Verification items for the finished model (mm, model axes). Face numbers are marked on the shaded views. A direction names the side the tool comes from. Coordinates: 2 decimals unless noted, no trailing zeros. Write each loop counter-clockwise with the first axis right and the second up, starting at its lowest first coordinate (ties: lowest second). Pieces come first, ordered by that corner, then holes. Notation, with made-up numbers: (-25, 23.25) - (28, 23.25) arc R26 ccw to (28, 62.25) - close; hole circle Ø2 at (14, 80). An arc over 180 degrees is marked (long way). Use CSV: the item, a comma, the result in double quotes. Start each with the question number.
```python
from build123d import *

# Parameters (mm, degrees)
F3_W          = 60
F3_H          = 91
F4_DEPTH      = 10
F5_W          = 56
F5_H          = 87
F6_DEPTH      = 8
F7_R          = 4
F8_DEPTH      = 10
F9_R          = 2
F10_DEPTH     = 10.001
F11_R         = 5
F12_R         = 5
F13_T1_DEPTH  = 77
F13_T3_DEPTH  = 14.5147186258
F13_T5_DEPTH  = 14.5147186258
F13_T8_ANGLE  = 90
F13_T10_ANGLE = 70.5287793655
F13_T12_ANGLE = 141.057558731
F13_T14_ANGLE = 90
F13_T16_ANGLE = 70.5287793655
F13_T18_ANGLE = 70.5287793655
F13_T20_ANGLE = 90
F13_T22_ANGLE = 141.057558731
F13_T24_ANGLE = 70.5287793655
F13_T26_ANGLE = 90
F13_T27_DEPTH = 81
F13_T29_DEPTH = 50
F13_T32_ANGLE = 90
F13_T34_ANGLE = 90
F13_T36_ANGLE = 90
F13_T38_ANGLE = 90


# Not quite as in the source:
# - a fillet or chamfer that OpenCascade refuses, or shapes differently, is made with other operations: its cross-section is extruded or revolved along the edge and cut away or added


with BuildPart() as f4:
    # F3 (on Top) → F4 (new body)
    with BuildSketch(Plane.XY):
        Rectangle(F3_W, F3_H)
    extrude(amount=F4_DEPTH)

    # F5 (on face) → F6 (cut)
    with BuildSketch(Plane.XY.offset(10)):
        Rectangle(F5_W, F5_H)
    extrude(amount=-F6_DEPTH, mode=Mode.SUBTRACT)

    # F7 (on face) → F8 (join)
    with BuildSketch(Plane(origin=(0, 0, 0), x_dir=(1, 0, 0), z_dir=(0, 0, -1))):
        with Locations((0, -41.5)):
            Circle(F7_R)
        with Locations((0, 41.5)):
            Circle(F7_R)
    extrude(amount=-F8_DEPTH)

    # F9 (on face) → F10 (cut, through all)
    with BuildSketch(Plane(origin=(0, 0, 0), x_dir=(1, 0, 0), z_dir=(0, 0, -1))):
        with Locations((0, -41.5)):
            Circle(F9_R)
        with Locations((0, 41.5)):
            Circle(F9_R)
    extrude(amount=-F10_DEPTH, mode=Mode.SUBTRACT)

    # F11
    f11_edges = [f4.edges().sort_by_distance(p)[0] for p in [
        (3.464102, 43.5, 6),
        (-3.464102, 43.5, 6),
        (-3.464102, -43.5, 6),
        (3.464102, -43.5, 6),
    ]]
    fillet(f11_edges, radius=F11_R)

    # F12
    f12_edges = [f4.edges().sort_by_distance(p)[0] for p in [
        (30, -45.5, 5),
        (-30, -45.5, 5),
        (30, 45.5, 5),
        (-30, 45.5, 5),
        (28, -43.5, 6),
        (-28, -43.5, 6),
        (-28, 43.5, 6),
        (28, 43.5, 6),
    ]]
    fillet(f12_edges, radius=F12_R)

    # F13: fillet of radius 3 on 24 edges, made by hand

    # F13_s2 → F13_t1 (join)
    with BuildSketch(Plane.XZ.offset(-38.5)):
        with BuildLine():
            ThreePointArc((-28, 5), (-27.1213203436, 2.8786796564), (-25, 2))
            Line((-25, 2), (-28, 2))
            Line((-28, 2), (-28, 5))
        make_face()
        with BuildLine():
            ThreePointArc((28, 5), (27.1213203436, 2.8786796564), (25, 2))
            Line((25, 2), (28, 2))
            Line((28, 2), (28, 5))
        make_face()
    extrude(amount=F13_T1_DEPTH)

    # F13_s4 → F13_t3 (join)
    with BuildSketch(Plane.YZ.offset(8.4852813742)):
        with BuildLine():
            ThreePointArc((-43.5, 5), (-42.6213203436, 2.8786796564), (-40.5, 2))
            Line((-40.5, 2), (-43.5, 2))
            Line((-43.5, 2), (-43.5, 5))
        make_face()
        with BuildLine():
            ThreePointArc((43.5, 5), (42.6213203436, 2.8786796564), (40.5, 2))
            Line((40.5, 2), (43.5, 2))
            Line((43.5, 2), (43.5, 5))
        make_face()
    extrude(amount=F13_T3_DEPTH)

    # F13_s6 → F13_t5 (join)
    with BuildSketch(Plane.YZ.offset(-23)):
        with BuildLine():
            ThreePointArc((-43.5, 5), (-42.6213203436, 2.8786796564), (-40.5, 2))
            Line((-40.5, 2), (-43.5, 2))
            Line((-43.5, 2), (-43.5, 5))
        make_face()
        with BuildLine():
            ThreePointArc((43.5, 5), (42.6213203436, 2.8786796564), (40.5, 2))
            Line((40.5, 2), (43.5, 2))
            Line((43.5, 2), (43.5, 5))
        make_face()
    extrude(amount=F13_T5_DEPTH)

    # F13_s7 → F13_t8 (revolve)
    with BuildSketch(Plane.YZ.offset(23)):
        with BuildLine():
            ThreePointArc((-43.5, 5), (-42.6213203436, 2.8786796564), (-40.5, 2))
            Line((-40.5, 2), (-43.5, 2))
            Line((-43.5, 2), (-43.5, 5))
        make_face()
    revolve(axis=Axis((23, -38.5, 2), (0, 0, 1)), revolution_arc=F13_T8_ANGLE)

    # F13_s9 → F13_t10 (revolve)
    with BuildSketch(Plane.YZ.offset(8.4852813742)):
        with BuildLine():
            ThreePointArc((-43.5, 5), (-42.6213203436, 2.8786796564), (-40.5, 2))
            Line((-40.5, 2), (-43.5, 2))
            Line((-43.5, 2), (-43.5, 5))
        make_face()
    revolve(axis=Axis((8.4852813742, -38.5, 2), (0, 0, -1)), revolution_arc=F13_T10_ANGLE)

    # F13_s11 → F13_t12 (revolve)
    with BuildSketch(Plane(origin=(-13.0421917419, -36.8888888889, 0), x_dir=(0, 0, 1), z_dir=(-0.3333333333, -0.9428090416, 0))):
        with BuildLine():
            ThreePointArc((5, -9.8333333333), (2.8786796564, -8.9546536769), (2, -6.8333333333))
            Line((2, -6.8333333333), (2, -9.8333333333))
            Line((2, -9.8333333333), (5, -9.8333333333))
        make_face()
    revolve(axis=Axis((0, -41.5, 2), (0, 0, -1)), revolution_arc=F13_T12_ANGLE)

    # F13_s13 → F13_t14 (revolve)
    with BuildSketch(Plane.XZ.offset(-38.5)):
        with BuildLine():
            ThreePointArc((28, 5), (27.1213203436, 2.8786796564), (25, 2))
            Line((25, 2), (28, 2))
            Line((28, 2), (28, 5))
        make_face()
    revolve(axis=Axis((23, 38.5, 2), (0, 0, 1)), revolution_arc=F13_T14_ANGLE)

    # F13_s15 → F13_t16 (revolve)
    with BuildSketch(Plane(origin=(-13.0421917419, -36.8888888889, 0), x_dir=(0, 0, 1), z_dir=(0.3333333333, 0.9428090416, 0))):
        with BuildLine():
            ThreePointArc((5, 9.8333333333), (2.8786796564, 8.9546536769), (2, 6.8333333333))
            Line((2, 6.8333333333), (2, 9.8333333333))
            Line((2, 9.8333333333), (5, 9.8333333333))
        make_face()
    revolve(axis=Axis((-8.4852813742, -38.5, 2), (0, 0, -1)), revolution_arc=F13_T16_ANGLE)

    # F13_s17 → F13_t18 (revolve)
    with BuildSketch(Plane.YZ.offset(8.4852813742)):
        with BuildLine():
            ThreePointArc((43.5, 5), (42.6213203436, 2.8786796564), (40.5, 2))
            Line((40.5, 2), (43.5, 2))
            Line((43.5, 2), (43.5, 5))
        make_face()
    revolve(axis=Axis((8.4852813742, 38.5, 2), (0, 0, 1)), revolution_arc=F13_T18_ANGLE)

    # F13_s19 → F13_t20 (revolve)
    with BuildSketch(Plane.YZ.offset(-23)):
        with BuildLine():
            ThreePointArc((-43.5, 5), (-42.6213203436, 2.8786796564), (-40.5, 2))
            Line((-40.5, 2), (-43.5, 2))
            Line((-43.5, 2), (-43.5, 5))
        make_face()
    revolve(axis=Axis((-23, -38.5, 2), (0, 0, -1)), revolution_arc=F13_T20_ANGLE)

    # F13_s21 → F13_t22 (revolve)
    with BuildSketch(Plane(origin=(13.0421917419, 36.8888888889, 0), x_dir=(0, 0, 1), z_dir=(0.3333333333, 0.9428090416, 0))):
        with BuildLine():
            ThreePointArc((5, -9.8333333333), (2.8786796564, -8.9546536769), (2, -6.8333333333))
            Line((2, -6.8333333333), (2, -9.8333333333))
            Line((2, -9.8333333333), (5, -9.8333333333))
        make_face()
    revolve(axis=Axis((0, 41.5, 2), (0, 0, -1)), revolution_arc=F13_T22_ANGLE)

    # F13_s23 → F13_t24 (revolve)
    with BuildSketch(Plane(origin=(-13.0421917419, 36.8888888889, 0), x_dir=(0, 0, 1), z_dir=(0.3333333333, -0.9428090416, 0))):
        with BuildLine():
            ThreePointArc((5, -9.8333333333), (2.8786796564, -8.9546536769), (2, -6.8333333333))
            Line((2, -6.8333333333), (2, -9.8333333333))
            Line((2, -9.8333333333), (5, -9.8333333333))
        make_face()
    revolve(axis=Axis((-8.4852813742, 38.5, 2), (0, 0, 1)), revolution_arc=F13_T24_ANGLE)

    # F13_s25 → F13_t26 (revolve)
    with BuildSketch(Plane.XZ.offset(-38.5)):
        with BuildLine():
            ThreePointArc((-28, 5), (-27.1213203436, 2.8786796564), (-25, 2))
            Line((-25, 2), (-28, 2))
            Line((-28, 2), (-28, 5))
        make_face()
    revolve(axis=Axis((-23, 38.5, 2), (0, 0, -1)), revolution_arc=F13_T26_ANGLE)

    # F13_s28 → F13_t27 (cut)
    with BuildSketch(Plane.XZ.offset(-40.5)):
        with BuildLine():
            ThreePointArc((30, 3), (29.1213203436, 0.8786796564), (27, 0))
            Line((27, 0), (30, 0))
            Line((30, 0), (30, 3))
        make_face()
        with BuildLine():
            ThreePointArc((-30, 3), (-29.1213203436, 0.8786796564), (-27, 0))
            Line((-27, 0), (-30, 0))
            Line((-30, 0), (-30, 3))
        make_face()
    extrude(amount=F13_T27_DEPTH, mode=Mode.SUBTRACT)

    # F13_s30 → F13_t29 (cut)
    with BuildSketch(Plane.YZ.offset(-25)):
        with BuildLine():
            ThreePointArc((-45.5, 3), (-44.6213203436, 0.8786796564), (-42.5, 0))
            Line((-42.5, 0), (-45.5, 0))
            Line((-45.5, 0), (-45.5, 3))
        make_face()
        with BuildLine():
            ThreePointArc((45.5, 3), (44.6213203436, 0.8786796564), (42.5, 0))
            Line((42.5, 0), (45.5, 0))
            Line((45.5, 0), (45.5, 3))
        make_face()
    extrude(amount=F13_T29_DEPTH, mode=Mode.SUBTRACT)

    # F13_s31 → F13_t32 (revolve, cut)
    with BuildSketch(Plane.YZ.offset(25)):
        with BuildLine():
            ThreePointArc((-45.5, 3), (-44.6213203436, 0.8786796564), (-42.5, 0))
            Line((-42.5, 0), (-45.5, 0))
            Line((-45.5, 0), (-45.5, 3))
        make_face()
    revolve(axis=Axis((25, -40.5, 0), (0, 0, 1)), revolution_arc=F13_T32_ANGLE, mode=Mode.SUBTRACT)

    # F13_s33 → F13_t34 (revolve, cut)
    with BuildSketch(Plane.YZ.offset(-25)):
        with BuildLine():
            ThreePointArc((-45.5, 3), (-44.6213203436, 0.8786796564), (-42.5, 0))
            Line((-42.5, 0), (-45.5, 0))
            Line((-45.5, 0), (-45.5, 3))
        make_face()
    revolve(axis=Axis((-25, -40.5, 0), (0, 0, -1)), revolution_arc=F13_T34_ANGLE, mode=Mode.SUBTRACT)

    # F13_s35 → F13_t36 (revolve, cut)
    with BuildSketch(Plane.XZ.offset(-40.5)):
        with BuildLine():
            ThreePointArc((30, 3), (29.1213203436, 0.8786796564), (27, 0))
            Line((27, 0), (30, 0))
            Line((30, 0), (30, 3))
        make_face()
    revolve(axis=Axis((25, 40.5, 0), (0, 0, 1)), revolution_arc=F13_T36_ANGLE, mode=Mode.SUBTRACT)

    # F13_s37 → F13_t38 (revolve, cut)
    with BuildSketch(Plane.XZ.offset(-40.5)):
        with BuildLine():
            ThreePointArc((-30, 3), (-29.1213203436, 0.8786796564), (-27, 0))
            Line((-27, 0), (-30, 0))
            Line((-30, 0), (-30, 3))
        make_face()
    revolve(axis=Axis((-25, 40.5, 0), (0, 0, -1)), revolution_arc=F13_T38_ANGLE, mode=Mode.SUBTRACT)


solid = f4.part
```
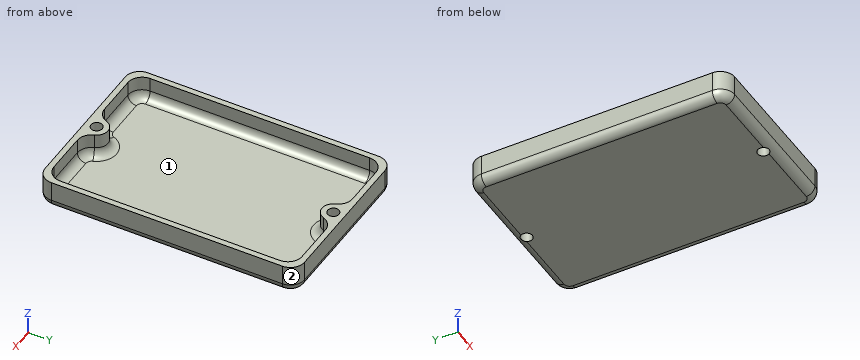
Q1. Cross-section at C-C (y = 18.5). Record the cut outline in (x, z), plus the area to 3 significant figures.
Q2. Cross-section at A-A (z = 8.25). Record the cut outline in (x, y).
Q3. Cross-section at B-B (x = -13). Record the cut outline in (y, z).
Q4. Gauge pin test, flat ends, axial feed: pin 1 (12 mm diameter, centred on x = 8, y = 21, fed in from +Z); pin 2 (10 mm diameter, centred on x = -22, y = -14, fed in from +Z); pin 3 (6.5 mm diameter, centred on x = 0, y = -41.5, fed in from -Z); pin 4 (2.5 mm diameter, centred on x = 0, y = 41.5, fed in from -Z). Record the tip position at first contact, or that the pin passes through.
Q5. Tool access check on the marked faces 1 and 2. Record the directions out of +Z, -Z, +X, -X, +Y, -Y that give a thin tool (end or side, any length) a straight path to the whole face; none if there is none.
Q6. Cross-section at D-D (x = 0). Record the cut outline in (y, z), plus the area to 3 significant figures.
Q7. Scan lines: line 1 along Y through (x, z) = (0, 5.75); line 2 along X through (y, z) = (29.5, 9.25); line 3 along Y through (x, z) = (16, 9.25). Record each from-to range of solid material in increasing order. Write a range as from..to.
Reply:
1,outline,"(-30, 3) arc R3 ccw to (-27, 0) - (27, 0) arc R3 ccw to (30, 3) - (30, 10) - (28, 10) - (28, 5) arc R3 cw to (25, 2) - (-25, 2) arc R3 cw to (-28, 5) - (-28, 10) - (-30, 10) - close"
1,area,"152 mm^2"
2,outline,"(-30, -40.5) arc R5 ccw to (-25, -45.5) - (25, -45.5) arc R5 ccw to (30, -40.5) - (30, 40.5) arc R5 ccw to (25, 45.5) - (-25, 45.5) arc R5 ccw to (-30, 40.5) - close; hole (-28, -38.5) arc R5 ccw to (-23, -43.5) - (-8.49, -43.5) arc R5 ccw to (-3.77, -40.17) arc R4 cw to (3.77, -40.17) arc R5 ccw to (8.49, -43.5) - (23, -43.5) arc R5 ccw to (28, -38.5) - (28, 38.5) arc R5 ccw to (23, 43.5) - (8.49, 43.5) arc R5 ccw to (3.77, 40.17) arc R4 cw to (-3.77, 40.17) arc R5 ccw to (-8.49, 43.5) - (-23, 43.5) arc R5 ccw to (-28, 38.5) - close; hole circle Ø4 at (0, -41.5); hole circle Ø4 at (0, 41.5)"
3,outline,"(-45.5, 3) arc R3 ccw to (-42.5, 0) - (42.5, 0) arc R3 ccw to (45.5, 3) - (45.5, 10) - (43.5, 10) - (43.5, 5) arc R3 cw to (40.5, 2) - (-40.5, 2) arc R3 cw to (-43.5, 5) - (-43.5, 10) - (-45.5, 10) - close"
4,pin 1,"z = 2"
4,pin 2,"z = 2.76"
4,pin 3,"z = 0"
4,pin 4,"through"
5,face 1,"+Z"
5,face 2,"+Z, -Z, +X, +Y"
6,outline,"(-45.5, 3) arc R3 ccw to (-43.5, 0.17) - (-43.5, 10) - (-45.5, 10) - close; (-39.5, 0) - (39.5, 0) - (39.5, 10) - (37.5, 10) - (37.5, 5) arc R3 cw to (34.5, 2) - (-34.5, 2) arc R3 cw to (-37.5, 5) - (-37.5, 10) - (-39.5, 10) - close; (43.5, 0.17) arc R3 ccw to (45.5, 3) - (45.5, 10) - (43.5, 10) - close"
6,area,"230 mm^2"
7,line 1,"-45.5..-43.5, -39.5..-37.5, 37.5..39.5, 43.5..45.5"
7,line 2,"-30..-28, 28..30"
7,line 3,"-45.5..-43.5, 43.5..45.5"
